```python
from build123d import *

# Parameters (mm, degrees)
STOCK_EXHAUST_M5_WASHER15_B_1_OUTLINE_R = 28
STOCK_EXHAUST_M5_WASHER15_B_1_DEPTH     = 20
SKETCH1_W                               = 20
SKETCH1_H                               = 20
CUT_EXTRUDE1_DEPTH                      = 3
LPATTERN1_COUNT                         = 2
LPATTERN1_PITCH                         = 25
LPATTERN1_COL_COUNT                     = 2
LPATTERN1_COL_PITCH                     = 25


# Read off the part's stored shape, not the designer's step: Stock-Exhaust_M5_washer15_B-1
with BuildPart() as part:
    # Stock-Exhaust_M5_washer15_B-1 outline → Stock-Exhaust_M5_washer15_B-1 (new body)
    with BuildSketch(Plane(origin=(0, 0, 0), x_dir=(1, 0, 0), z_dir=(0, 1, 0))):
        with BuildLine():
            Line((200, -15), (135, -15))
            Line((135, -15), (135, -10))
            Line((135, -10), (200, -10))
            Line((200, -10), (200, 10))
            Line((200, 10), (135, 10))
            Line((135, 10), (135, 15))
            Line((135, 15), (200, 15))
            Line((200, 15), (200, 35))
            Line((200, 35), (28.284271247, 35))
            ThreePointArc((28.284271247, 35), (-45, 0), (28.284271247, -35))
            Line((28.284271247, -35), (200, -35))
            Line((200, -35), (200, -15))
        make_face()
        with BuildLine():
            ThreePointArc((52.915026221, -15), (53.557527969, -12.513640473), (54.083269132, -10))
            Line((54.083269132, -10), (115, -10))
            Line((115, -10), (115, -15))
            Line((115, -15), (52.915026221, -15))
        make_face(mode=Mode.SUBTRACT)
        Circle(STOCK_EXHAUST_M5_WASHER15_B_1_OUTLINE_R, mode=Mode.SUBTRACT)
        with BuildLine():
            ThreePointArc((54.083269132, 10), (53.557527969, 12.513640473), (52.915026221, 15))
            Line((52.915026221, 15), (115, 15))
            Line((115, 15), (115, 10))
            Line((115, 10), (54.083269132, 10))
        make_face(mode=Mode.SUBTRACT)
    extrude(amount=STOCK_EXHAUST_M5_WASHER15_B_1_DEPTH)

    # Sketch1 → Cut-Extrude1 (cut)
    with BuildSketch(Plane(origin=(200, 0, 0), x_dir=(0, 0, -1), z_dir=(1, 0, 0))):
        with Locations((0, 10)):
            Rectangle(SKETCH1_W, SKETCH1_H)
    cut_extrude1 = extrude(amount=-CUT_EXTRUDE1_DEPTH, mode=Mode.SUBTRACT)

    # LPattern1: Cut-Extrude1 ×2
    with Locations(*[(0, 0, -i * LPATTERN1_PITCH) for i in range(1, LPATTERN1_COUNT)]):
        add(cut_extrude1, mode=Mode.SUBTRACT)

    # LPattern1 col: Cut-Extrude1 ×2
    with Locations(*[(0, 0, i * LPATTERN1_COL_PITCH) for i in range(1, LPATTERN1_COL_COUNT)]):
        add(cut_extrude1, mode=Mode.SUBTRACT)


solid = part.part
```
CAD build for the part. Positions are in the model's coordinates, mm. A direction names the side the tool comes from. Round coordinates to 2 decimals unless told otherwise and drop trailing zeros. Loops run counter-clockwise (first coordinate to the right, second up) from the corner with the lowest first, then second, coordinate; pieces in that order, holes last. Notation, with made-up numbers: M 58.5,-20 L 63.5,-20 A20 cw 63.5,-3 Z; hole C 6,82.25 d5. An arc over 180 degrees is marked long. Return JSON: item names as keys, results as strings. Group by question number.
(1) Saw through at C-C, the plane y = 2.25. List the corners of the cut face in (x, z), and give its area (3 significant figures).
(2) Saw through at A-A, the plane x = 153. List the corners of the cut face in (y, z), and give its area (3 significant figures).
(3) Drop flat-ended pins along their axis: P1, Ø2, axis at x = 34.5, y = 6.5, coming from the +Z side; P2, Ø2, axis at x = 16.5, y = 14, coming from the -Z side; P3, Ø1.5, axis at y = 9.5, z = 11.5, coming from the -X side. Give the stop position or say it passes through.
(4) Saw through at B-B, the plane z = 0. List the corners of the cut face in (x, y).
(5) Wall check: probe 1 along Z at (x, y) = (156.5, 5.25); probe 2 along X at (y, z) = (5.75, 13); probe 3 along Z at (x, y) = (0, 8.5). Give the ranges that are in metal, low to high. Write a range as [from, to].
(6) Tool access for faces 4 (the flat face through (84, 10, 15)), 5 (the flat face through (166, 10, 10)), 6 (the flat face through (114, 10, -35)), 7 (the flat face through (197, 10, -25)): list every direction of +Z, -Z, +X, -X, +Y, -Y with a clear straight run to the whole face (end or side of a thin tool).
(7) Mould opens along Z. For faces 1 (the flat face through (74, 20, -1)), 2 (the flat face through (111, 10, 35)), 3 (the flat face through (135, 10, -12)) say: +Z half, -Z half, draft (parallel to the pull), parting line (faces both ways), or undercut.
(8) Saw through at D-D, the plane x = 0. List the corners of the cut face in (y, z).
Answer list:
{
 "1": {"outline": "M 28.28,-35 L 197,-35 L 197,-15 L 135,-15 L 135,-10 L 197,-10 L 197,10 L 135,10 L 135,15 L 197,15 L 197,35 L 28.28,35 A45 ccw long Z; hole C 0,0 d56; hole M 52.92,-15 L 115,-15 L 115,-10 L 54.08,-10 A55 cw Z; hole M 52.92,15 A55 cw 54.08,10 L 115,10 L 115,15 Z", "area": "13,700 mm2"},
 "2": {"outline": "M 0,-35 L 20,-35 L 20,-15 L 0,-15 Z; M 0,-10 L 20,-10 L 20,10 L 0,10 Z; M 0,15 L 20,15 L 20,35 L 0,35 Z", "area": "1,200 mm2"},
 "3": {"P1": "z = 35", "P2": "z = -42.25", "P3": "x = -43.7"},
 "4": {"outline": "M -45,0 L -28,0 L -28,20 L -45,20 Z; M 28,0 L 197,0 L 197,20 L 28,20 Z"},
 "5": {"probe 1": "[-35, -15], [-10, 10], [15, 35]", "probe 2": "[-43.08, -24.8], [24.8, 53.44], [115, 135]", "probe 3": "[-45, -28], [28, 45]"},
 "6": {"face 4": "+Y, -Y", "face 5": "+X, +Y, -Y", "face 6": "-Z, +X, +Y, -Y", "face 7": "+Z, -Z, +X, +Y, -Y"},
 "7": {"face 1": "draft", "face 2": "+Z half", "face 3": "undercut"},
 "8": {"outline": "M 0,-45 L 20,-45 L 20,-28 L 0,-28 Z; M 0,28 L 20,28 L 20,45 L 0,45 Z"}
}
